Part model, mm, in its own coordinate system. Round coordinates to 2 decimals unless told otherwise and drop trailing zeros. Write each loop counter-clockwise with the first axis right and the second up, starting at its lowest first coordinate (ties: lowest second). Pieces come first, ordered by that corner, then holes.
```python
from build123d import *

# Parameters (mm, degrees)
BOSS_EXTRUDE1_DEPTH = 40
FILLET3_R           = 20
FILLET4_R           = 20
SKETCH2_R           = 5
SKETCH2_R_2         = 2.5
CUT_EXTRUDE1_DEPTH  = 5
SKETCH3_R           = 5
CUT_EXTRUDE2_DEPTH  = 5


with BuildPart() as part:
    # Sketch1 → Boss-Extrude1 (new body)
    with BuildSketch(Plane(origin=(0, 0, 0), x_dir=(0, 0, -1), z_dir=(1, 0, 0))):
        with BuildLine():
            Line((-58.598472687, -15.960552102), (-57.184259125, -14.54633854))
            Line((-57.184259125, -14.54633854), (-34.253623627, 8.384296958))
            Line((-34.253623627, 8.384296958), (81.408669988, 124.046590573))
            ThreePointArc((81.408669988, 124.046590573), (81.994456425, 125.460804135), (81.408669988, 126.875017697))
            Line((81.408669988, 126.875017697), (80.703876553, 127.579811132))
            ThreePointArc((80.703876553, 127.579811132), (79.289662991, 128.165597569), (77.875449429, 127.579811132))
            Line((77.875449429, 127.579811132), (-37.786844186, 11.917517517))
            Line((-37.786844186, 11.917517517), (-60.717479684, -11.013117981))
            Line((-60.717479684, -11.013117981), (-62.131693246, -12.427331543))
            Line((-62.131693246, -12.427331543), (-60.717479684, -13.841545106))
            Line((-60.717479684, -13.841545106), (-60.01268625, -14.54633854))
            Line((-60.01268625, -14.54633854), (-58.598472687, -15.960552102))
        make_face()
    extrude(amount=BOSS_EXTRUDE1_DEPTH)

    # Fillet3
    fillet3_edges = [part.edges().sort_by_distance(p)[0] for p in [
        (40, -14.193941823, 60.365082967),
    ]]
    fillet(fillet3_edges, radius=FILLET3_R)

    # Fillet4
    fillet4_edges = [part.edges().sort_by_distance(p)[0] for p in [
        (0, -14.193941823, 60.365082967),
    ]]
    fillet(fillet4_edges, radius=FILLET4_R - 0.0001)  # a hair under: the kernel refuses the full size

    # Sketch2 → Cut-Extrude1 (cut)
    with BuildSketch(Plane(origin=(0, 24.852180852, 24.852180852), x_dir=(1, 0, 0), z_dir=(0, 0.7071067811865465, 0.7071067811865487))):
        with Locations(Location((20, -32.721192027, 0), (0, 0, 270))):
            Circle(SKETCH2_R)
        with Locations(Location((35, 100.778807973, 0), (0, 0, 270))):
            Circle(SKETCH2_R_2)
        with Locations(Location((35, 56.278807973, 0), (0, 0, 270))):
            Circle(SKETCH2_R_2)
        with Locations(Location((35, 11.778807973, 0), (0, 0, 270))):
            Circle(SKETCH2_R_2)
        with Locations(Location((5, 11.778807973, 0), (0, 0, 90))):
            Circle(SKETCH2_R_2)
        with Locations(Location((5, 56.278807973, 0), (0, 0, 90))):
            Circle(SKETCH2_R_2)
        with Locations(Location((5, 100.778807973, 0), (0, 0, 90))):
            Circle(SKETCH2_R_2)
    extrude(amount=-CUT_EXTRUDE1_DEPTH, mode=Mode.SUBTRACT)

    # Sketch3 → Cut-Extrude2 (cut)
    with BuildSketch(Plane(origin=(0, 21.318960292, 21.318960292), x_dir=(1, 0, 0), z_dir=(0, -0.7071067811865434, -0.7071067811865518))):
        with Locations(Location((20, -133.888702436, 0), (0, 0, 270))):
            Circle(SKETCH3_R)
    extrude(amount=-CUT_EXTRUDE2_DEPTH, mode=Mode.SUBTRACT)


solid = part.part
```
Q1. Wall check: L1, parallel to Z at x = 24.5, y = 52; L2, parallel to Y at x = 25, z = -44.5; L3, parallel to Z at x = 18.5, y = 46. Give the ranges that are in metal, low to high.
Values follow:
L1: z = -9.36 to -2.3
L2: y = 87.14 to 94.2
L3: z = -3.36 to 3.7
Q2. Cut at B-B on y = 17. Write the cut outline in (x, z).
Values follow:
outline: (0, 25.64) - (40, 25.64) - (40, 32.7) - (0, 32.7) - close
Q3. Mould opens along Z. For faces 1 (the flat face through (19.72, 58.556, -8.852)), 2 (the flat face through (19.72, 53.063, -10.425)), 3 (the cylindrical face through (4.25, 33.13, 13.1)) say: +Z half, -Z half, draft (parallel to the pull), parting line (faces both ways), or undercut.
Values follow:
face 1: +Z half
face 2: -Z half
face 3: undercut
Q4. Cut at A-A on x = 18. Write the cut outline in (y, z).
Values follow:
outline: (-15.89, 58.53) - (-5.06, 47.7) - (-1.53, 51.23) - (-12.36, 62.06) - close; (1.42, 41.22) - (112.75, -70.11) - (116.29, -66.58) - (4.96, 44.75) - close; (119.23, -76.6) - (124.05, -81.41) arc R2 ccw to (126.88, -81.41) - (127.58, -80.7) arc R2 ccw to (127.58, -77.88) - (122.77, -73.06) - close
Q5. Cut at C-C on z = -28. Write the cut outline in (x, y), plus the area to 3 significant figures.
Values follow:
outline: (0, 70.64) - (40, 70.64) - (40, 77.7) - (0, 77.7) - close
area: 283 mm2
Q6. Drop flat-ended pins along their axis: pin 1 (3 mm diameter, centred on x = 30.5, y = 86, fed in from +Z); pin 2 (1 mm diameter, centred on x = 10.5, z = -20, fed in from +Y); pin 3 (10 mm diameter, centred on x = 6.5, z = -29.5, fed in from +Y). Give the stop position or say it passes through.
Values follow:
pin 1: stops at z = -34.8
pin 2: stops at y = 70.2
pin 3: stops at y = 84.2
